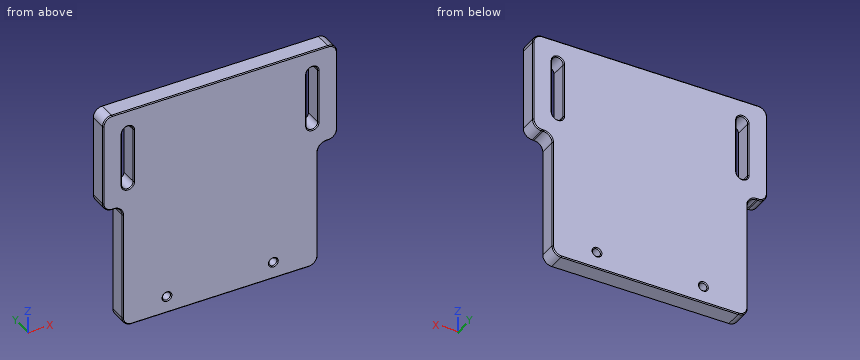
from build123d import *

# Parameters (mm, degrees)
SKETCH1_W                 = 66
SKETCH1_H                 = 63.5
BOSS_EXTRUDE1_DEPTH       = 5.08
SKETCH6_W                 = 5.5
SKETCH6_H                 = 35.589114281
CUT_EXTRUDE1_DEPTH        = 5.08
F_4_40_TAPPED_HOLE1_D     = 2.2606
F_4_40_TAPPED_HOLE1_DEPTH = 7.5946
F_4_40_TAPPED_HOLE1_TIP   = 0.679152758
FILLET1_R                 = 2.54
FILLET2_R                 = 2.54
CUT_EXTRUDE2_DEPTH        = 6.08
CHAMFER1_SIZE             = 0.254


with BuildPart() as part:
    # Sketch1 → Boss-Extrude1 (new body)
    with BuildSketch(Plane(origin=(0, 0, 0), x_dir=(1, 0, 0), z_dir=(0, 1, 0))):
        with Locations((-33, 31.75)):
            Rectangle(SKETCH1_W, SKETCH1_H)
    extrude(amount=BOSS_EXTRUDE1_DEPTH)

    # Sketch6 → Cut-Extrude1 (cut)
    with BuildSketch(Plane(origin=(0, 5.08, 0), x_dir=(1, 0, 0), z_dir=(0, 1, 0))):
        with Locations((-63.25, 45.70544286)):
            Rectangle(SKETCH6_W, SKETCH6_H)
        with Locations((-2.75, 45.70544286)):
            Rectangle(SKETCH6_W, SKETCH6_H)
    extrude(amount=-CUT_EXTRUDE1_DEPTH, mode=Mode.SUBTRACT)

    # #4-40 Tapped Hole1
    with Locations(Plane(origin=(0, 5.08, 0), x_dir=(-1, 0, 0), z_dir=(0, 1, 0))):
        with Locations((48, -58.7375), (18, -58.7375)):
            Hole(F_4_40_TAPPED_HOLE1_D / 2, depth=F_4_40_TAPPED_HOLE1_DEPTH)
            with Locations((0, 0, -(F_4_40_TAPPED_HOLE1_DEPTH + F_4_40_TAPPED_HOLE1_TIP / 2))):  # 118° drill point
                Cone(0, F_4_40_TAPPED_HOLE1_D / 2, F_4_40_TAPPED_HOLE1_TIP, mode=Mode.SUBTRACT)

    # Fillet1
    fillet1_edges = [part.edges().sort_by_distance(p)[0] for p in [
        (-60.5, 2.54, -63.5),
        (-60.5, 2.54, -27.910885719),
        (-5.5, 2.54, -27.910885719),
        (-5.5, 2.54, -63.5),
        (0, 2.54, 0),
        (-66, 2.54, 0),
    ]]
    fillet(fillet1_edges, radius=FILLET1_R)

    # Fillet2
    fillet2_edges = [part.edges().sort_by_distance(p)[0] for p in [
        (-66, 2.54, -27.910885719),
        (0, 2.54, -27.910885719),
    ]]
    fillet(fillet2_edges, radius=FILLET2_R)

    # Sketch9 → Cut-Extrude2 (cut, through all)
    with BuildSketch(Plane(origin=(0, 5.08, 0), x_dir=(1, 0, 0), z_dir=(0, 1, 0))):
        with BuildLine():
            Line((-60.6383, 6.35), (-60.6383, 21.59))
            ThreePointArc((-60.6383, 21.59), (-59, 23.2283), (-57.3617, 21.59))
            Line((-57.3617, 21.59), (-57.3617, 6.35))
            ThreePointArc((-57.3617, 6.35), (-59, 4.7117), (-60.6383, 6.35))
        make_face()
        with BuildLine():
            Line((-8.6383, 6.35), (-8.6383, 21.59))
            ThreePointArc((-8.6383, 21.59), (-7, 23.2283), (-5.3617, 21.59))
            Line((-5.3617, 21.59), (-5.3617, 6.35))
            ThreePointArc((-5.3617, 6.35), (-7, 4.7117), (-8.6383, 6.35))
        make_face()
    extrude(amount=-CUT_EXTRUDE2_DEPTH, mode=Mode.SUBTRACT)

    # Chamfer1
    chamfer1_edges = [part.edges().sort_by_distance(p)[0] for p in [
        (-59, 0, -4.7117),
        (-60.6383, 0, -13.97),
        (-59, 0, -23.2283),
        (-57.3617, 0, -13.97),
        (-59, 5.08, -4.7117),
        (-57.3617, 5.08, -13.97),
        (-59, 5.08, -23.2283),
        (-60.6383, 5.08, -13.97),
        (-7, 0, -4.7117),
        (-8.6383, 0, -13.97),
        (-7, 0, -23.2283),
        (-5.3617, 0, -13.97),
        (-7, 5.08, -4.7117),
        (-5.3617, 5.08, -13.97),
        (-7, 5.08, -23.2283),
        (-8.6383, 5.08, -13.97),
        (-19.1303, 0, -58.7375),
        (-19.1303, 5.08, -58.7375),
        (-49.1303, 0, -58.7375),
        (-49.1303, 5.08, -58.7375),
        (-33, 0, 0),
        (-33, 5.08, 0),
        (-5.5, 0, -45.705442859),
        (-2.75, 0, -27.910885719),
        (0, 0, -13.955442859),
        (-60.5, 0, -45.705442859),
        (-33, 0, -63.5),
        (-59.756051224, 0, -62.756051224),
        (-6.243948776, 0, -62.756051224),
        (-0.743948776, 0, -0.743948776),
        (-65.256051224, 0, -0.743948776),
        (-2.75, 5.08, -27.910885719),
        (-5.5, 5.08, -45.705442859),
        (-33, 5.08, -63.5),
        (-60.5, 5.08, -45.705442859),
        (0, 5.08, -13.955442859),
        (-59.756051224, 5.08, -62.756051224),
        (-6.243948776, 5.08, -62.756051224),
        (-0.743948776, 5.08, -0.743948776),
        (-65.256051224, 5.08, -0.743948776),
        (-4.756051224, 5.08, -28.654834495),
        (-4.756051224, 0, -28.654834495),
        (-61.243948776, 5.08, -28.654834495),
        (-61.243948776, 0, -28.654834495),
        (-63.25, 5.08, -27.910885719),
        (-63.25, 0, -27.910885719),
        (-66, 5.08, -13.955442859),
        (-0.743948776, 5.08, -27.166936943),
        (-65.256051224, 5.08, -27.166936943),
        (-66, 0, -13.955442859),
        (-0.743948776, 0, -27.166936943),
        (-65.256051224, 0, -27.166936943),
    ]]
    chamfer(chamfer1_edges, length=CHAMFER1_SIZE)


solid = part.part
For this review, take the finished solid that the model builds, in its own axes (mm). Coordinates: 2 decimals unless noted, no trailing zeros. Order: outer loops, then holes, each group sorted by start corner. A loop starts at its lowest first (then second) coordinate and runs counter-clockwise, first axis right, second up. Notation, with made-up numbers: (50.25, 71) - (87.25, 71) arc R14 cw to (87.25, 95) - close; hole circle Ø9 at (32.25, 83.5). An arc over 180 degrees is marked (long way). Answer as CSV lines item,"result". Start each with the question number.
1) Add section C-C (y = 3.9). State the section outline as (x, z) points.
2) Add section D-D (z = -43). State the section outline as (x, y) points, then the cut area to 3 significant figures.
3) Add section B-B (z = -12). State the section outline as (x, y) points.
4) To check wall thickness, follow line 1 along X through (y, z) = (3.1, -8.5); line 2 along Z through (x, y) = (-18, 1.3); line 3 along Z through (x, y) = (-8.5, 1.3). State the ranges of each line that lie inside material, in increasing order. Write a range as [from, to].
5) Add section A-A (x = -48). State the section outline as (y, z) points.
6) Insertion check: P1, Ø2.5, axis at x = -18, z = -58.74, coming from the +Y side; P2, Ø2, axis at y = 4, z = -29.5, coming from the -X side; P3, Ø2, axis at y = 2, z = -48, coming from the +X side. Each pin has a flat end and moves straight along its axis. Give the tip position at first contact, or say it passes through.
Result:
1,outline,"(-66, -25.37) arc R2.54 ccw to (-63.46, -27.91) - (-63.04, -27.91) arc R2.54 cw to (-60.5, -30.45) - (-60.5, -60.96) arc R2.54 ccw to (-57.96, -63.5) - (-8.04, -63.5) arc R2.54 ccw to (-5.5, -60.96) - (-5.5, -30.45) arc R2.54 cw to (-2.96, -27.91) - (-2.54, -27.91) arc R2.54 ccw to (0, -25.37) - (0, -2.54) arc R2.54 ccw to (-2.54, 0) - (-63.46, 0) arc R2.54 ccw to (-66, -2.54) - close; hole (-60.64, -21.59) arc R1.64 ccw to (-57.36, -21.59) - (-57.36, -6.35) arc R1.64 ccw to (-60.64, -6.35) - close; hole circle Ø2.26 at (-48, -58.74); hole circle Ø2.26 at (-18, -58.74); hole (-8.64, -21.59) arc R1.64 ccw to (-5.36, -21.59) - (-5.36, -6.35) arc R1.64 ccw to (-8.64, -6.35) - close"
2,outline,"(-60.5, 0.25) - (-60.25, 0) - (-5.75, 0) - (-5.5, 0.25) - (-5.5, 4.83) - (-5.75, 5.08) - (-60.25, 5.08) - (-60.5, 4.83) - close"
2,area,"279 mm^2"
3,outline,"(-66, 0.25) - (-65.75, 0) - (-60.89, 0) - (-60.64, 0.25) - (-60.64, 4.83) - (-60.89, 5.08) - (-65.75, 5.08) - (-66, 4.83) - close; (-57.36, 0.25) - (-57.11, 0) - (-8.89, 0) - (-8.64, 0.25) - (-8.64, 4.83) - (-8.89, 5.08) - (-57.11, 5.08) - (-57.36, 4.83) - close; (-5.36, 0.25) - (-5.11, 0) - (-0.25, 0) - (0, 0.25) - (0, 4.83) - (-0.25, 5.08) - (-5.11, 5.08) - (-5.36, 4.83) - close"
4,line 1,"[-66, -60.64], [-57.36, -8.64], [-5.36, 0]"
4,line 2,"[-63.5, -59.87], [-57.61, 0]"
4,line 3,"[-63.5, -22.25], [-5.69, 0]"
5,outline,"(0, -63.25) - (0.25, -63.5) - (4.83, -63.5) - (5.08, -63.25) - (5.08, -60.12) - (4.83, -59.87) - (0.25, -59.87) - (0, -60.12) - close; (0, -57.35) - (0.25, -57.61) - (4.83, -57.61) - (5.08, -57.35) - (5.08, -0.25) - (4.83, 0) - (0.25, 0) - (0, -0.25) - close"
6,P1,"y = 4.95"
6,P2,"x = -61.41"
6,P3,"x = -5.5"
